For this review, take the finished solid that the model builds, in its own axes (mm). Face numbers are marked on the shaded views. A direction names the side the tool comes from. Give positions to 0.01 mm unless a question says otherwise; leave off trailing zeros. Order: outer loops, then holes, each group sorted by start corner. A loop starts at its lowest first (then second) coordinate and runs counter-clockwise, first axis right, second up. Notation, with made-up numbers: (-27, 65) - (9, 65) arc R15 ccw to (9, 85) - close; hole circle Ø5 at (43.5, 7.25). An arc over 180 degrees is marked (long way). Answer as a JSON object with one key per item and string values. Group by question number.
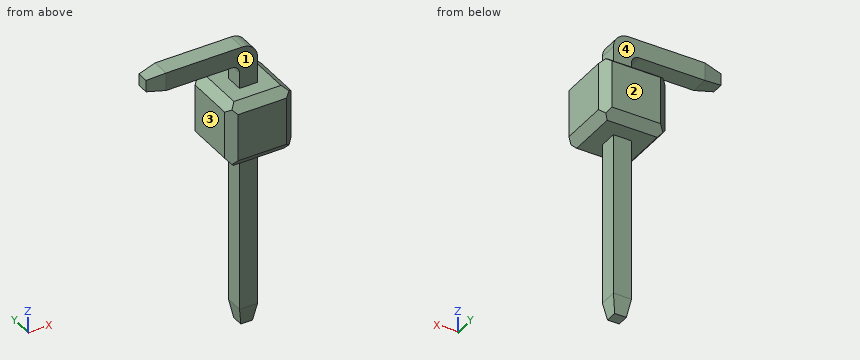
from build123d import *
from OCP.BRepFilletAPI import BRepFilletAPI_MakeChamfer

# Parameters (mm, degrees)
EXTRUDE_1_DEPTH = 0.7
CHAMFER_1_SIZE  = 0.7
CHAMFER_1_SIZE2 = 0.123428886
CHAMFER_2_SIZE  = 0.7
CHAMFER_2_SIZE2 = 0.123428886
SKETCH_2_W      = 2.54
SKETCH_2_H      = 2.54
EXTRUDE_2_DEPTH = 2.5
CHAMFER_3_SIZE  = 0.3
CHAMFER_3_SIZE2 = 0.357526078
CHAMFER_4_SIZE  = 0.3
CHAMFER_4_SIZE2 = 0.357526078
CHAMFER_5_SIZE  = 0.3
CHAMFER_5_SIZE2 = 0.357526078


with BuildPart() as part:
    # Эскиз1 → Бобышка-Вытянуть1 (new body)
    with BuildSketch(Plane(origin=(0, 0, 0), x_dir=(1, 0, 0), z_dir=(0, 1, 0))):
        with BuildLine():
            Line((0.35, 0), (0.35, -10.55))
            ThreePointArc((0.35, -10.55), (0.174264069, -10.974264069), (-0.25, -11.15))
            Line((-0.25, -11.15), (-3.9, -11.15))
            Line((-3.9, -11.15), (-3.9, -10.45))
            Line((-3.9, -10.45), (-0.65, -10.45))
            ThreePointArc((-0.65, -10.45), (-0.437867966, -10.362132034), (-0.35, -10.15))
            Line((-0.35, -10.15), (-0.35, 0))
            Line((-0.35, 0), (0.35, 0))
        make_face()
    extrude(amount=EXTRUDE_1_DEPTH)

    # Фаска1: one chamfer whose edges measure the first distance from different faces: ONE call of the kernel's chamfer builder (chamfer() names one face for all edges)
    chamfer_1_edges_1 = [part.edges().sort_by_distance(p)[0] for p in [
        (0, 0, 0),
    ]]
    chamfer_1_side_1 = [part.faces().sort_by_distance(p)[0] for p in [
        (-0.230674814, 0, 5.075),
    ]]
    chamfer_1_edges_2 = [part.edges().sort_by_distance(p)[0] for p in [
        (0.35, 0.35, 0),
    ]]
    chamfer_1_side_2 = [part.faces().sort_by_distance(p)[0] for p in [
        (0.35, 0.35, 5.275),
    ]]
    chamfer_1_edges_3 = [part.edges().sort_by_distance(p)[0] for p in [
        (-0.35, 0.35, 0),
    ]]
    chamfer_1_side_3 = [part.faces().sort_by_distance(p)[0] for p in [
        (-0.35, 0.35, 5.075),
    ]]
    chamfer_1_edges_4 = [part.edges().sort_by_distance(p)[0] for p in [
        (0, 0.7, 0),
    ]]
    chamfer_1_side_4 = [part.faces().sort_by_distance(p)[0] for p in [
        (-0.230674814, 0.7, 5.075),
    ]]
    chamfer_1 = BRepFilletAPI_MakeChamfer(part.part.solid().wrapped)
    for e in chamfer_1_edges_1:
        chamfer_1.Add(CHAMFER_1_SIZE, CHAMFER_1_SIZE2, e.wrapped, chamfer_1_side_1[0].wrapped)  # the first distance lies on this face
    for e in chamfer_1_edges_2:
        chamfer_1.Add(CHAMFER_1_SIZE, CHAMFER_1_SIZE2, e.wrapped, chamfer_1_side_2[0].wrapped)  # the first distance lies on this face
    for e in chamfer_1_edges_3:
        chamfer_1.Add(CHAMFER_1_SIZE, CHAMFER_1_SIZE2, e.wrapped, chamfer_1_side_3[0].wrapped)  # the first distance lies on this face
    for e in chamfer_1_edges_4:
        chamfer_1.Add(CHAMFER_1_SIZE, CHAMFER_1_SIZE2, e.wrapped, chamfer_1_side_4[0].wrapped)  # the first distance lies on this face
    add(Compound.cast(chamfer_1.Shape()), mode=Mode.REPLACE)

    # Фаска2: one chamfer whose edges measure the first distance from different faces: ONE call of the kernel's chamfer builder (chamfer() names one face for all edges)
    chamfer_2_edges_1 = [part.edges().sort_by_distance(p)[0] for p in [
        (-3.9, 0.35, 11.15),
    ]]
    chamfer_2_side_1 = [part.faces().sort_by_distance(p)[0] for p in [
        (-2.075, 0.35, 11.15),
    ]]
    chamfer_2_edges_2 = [part.edges().sort_by_distance(p)[0] for p in [
        (-3.9, 0.35, 10.45),
    ]]
    chamfer_2_side_2 = [part.faces().sort_by_distance(p)[0] for p in [
        (-2.275, 0.35, 10.45),
    ]]
    chamfer_2_edges_3 = [part.edges().sort_by_distance(p)[0] for p in [
        (-3.9, 0.7, 10.8),
    ]]
    chamfer_2_side_3 = [part.faces().sort_by_distance(p)[0] for p in [
        (-0.23718821, 0.7, 5.425),
    ]]
    chamfer_2_edges_4 = [part.edges().sort_by_distance(p)[0] for p in [
        (-3.9, 0, 10.8),
    ]]
    chamfer_2_side_4 = [part.faces().sort_by_distance(p)[0] for p in [
        (-0.23718821, 0, 5.425),
    ]]
    chamfer_2 = BRepFilletAPI_MakeChamfer(part.part.solid().wrapped)
    for e in chamfer_2_edges_1:
        chamfer_2.Add(CHAMFER_2_SIZE, CHAMFER_2_SIZE2, e.wrapped, chamfer_2_side_1[0].wrapped)  # the first distance lies on this face
    for e in chamfer_2_edges_2:
        chamfer_2.Add(CHAMFER_2_SIZE, CHAMFER_2_SIZE2, e.wrapped, chamfer_2_side_2[0].wrapped)  # the first distance lies on this face
    for e in chamfer_2_edges_3:
        chamfer_2.Add(CHAMFER_2_SIZE, CHAMFER_2_SIZE2, e.wrapped, chamfer_2_side_3[0].wrapped)  # the first distance lies on this face
    for e in chamfer_2_edges_4:
        chamfer_2.Add(CHAMFER_2_SIZE, CHAMFER_2_SIZE2, e.wrapped, chamfer_2_side_4[0].wrapped)  # the first distance lies on this face
    add(Compound.cast(chamfer_2.Shape()), mode=Mode.REPLACE)

    # Эскиз2 → Бобышка-Вытянуть2 (add)
    with BuildSketch(Plane.XY.offset(9.53)):
        with Locations((0, 0.35)):
            Rectangle(SKETCH_2_W, SKETCH_2_H)
    extrude(amount=-EXTRUDE_2_DEPTH)

    # Фаска3
    chamfer_3_edges = [part.edges().sort_by_distance(p)[0] for p in [
        (-1.27, 0.35, 7.03),
        (0, 1.62, 7.03),
        (1.27, 0.35, 7.03),
        (0, -0.92, 7.03),
    ]]
    chamfer_3_side = [part.faces().sort_by_distance(p)[0] for p in [
        (0, -0.884078976, 7.03),
    ]]
    chamfer(chamfer_3_edges, length=CHAMFER_3_SIZE, length2=CHAMFER_3_SIZE2, reference=chamfer_3_side[0])

    # Фаска4: one chamfer whose edges measure the first distance from different faces: ONE call of the kernel's chamfer builder (chamfer() names one face for all edges)
    chamfer_4_edges_1 = [part.edges().sort_by_distance(p)[0] for p in [
        (-1.27, 0.35, 9.53),
    ]]
    chamfer_4_side_1 = [part.faces().sort_by_distance(p)[0] for p in [
        (-1.27, 0.35, 8.458763039),
    ]]
    chamfer_4_edges_2 = [part.edges().sort_by_distance(p)[0] for p in [
        (0, -0.92, 9.53),
    ]]
    chamfer_4_side_2 = [part.faces().sort_by_distance(p)[0] for p in [
        (0, -0.92, 8.458763039),
    ]]
    chamfer_4_edges_3 = [part.edges().sort_by_distance(p)[0] for p in [
        (1.27, 0.35, 9.53),
    ]]
    chamfer_4_side_3 = [part.faces().sort_by_distance(p)[0] for p in [
        (1.27, 0.35, 8.458763039),
    ]]
    chamfer_4_edges_4 = [part.edges().sort_by_distance(p)[0] for p in [
        (0, 1.62, 9.53),
    ]]
    chamfer_4_side_4 = [part.faces().sort_by_distance(p)[0] for p in [
        (0, 1.62, 8.458763039),
    ]]
    chamfer_4 = BRepFilletAPI_MakeChamfer(part.part.solid().wrapped)
    for e in chamfer_4_edges_1:
        chamfer_4.Add(CHAMFER_4_SIZE, CHAMFER_4_SIZE2, e.wrapped, chamfer_4_side_1[0].wrapped)  # the first distance lies on this face
    for e in chamfer_4_edges_2:
        chamfer_4.Add(CHAMFER_4_SIZE, CHAMFER_4_SIZE2, e.wrapped, chamfer_4_side_2[0].wrapped)  # the first distance lies on this face
    for e in chamfer_4_edges_3:
        chamfer_4.Add(CHAMFER_4_SIZE, CHAMFER_4_SIZE2, e.wrapped, chamfer_4_side_3[0].wrapped)  # the first distance lies on this face
    for e in chamfer_4_edges_4:
        chamfer_4.Add(CHAMFER_4_SIZE, CHAMFER_4_SIZE2, e.wrapped, chamfer_4_side_4[0].wrapped)  # the first distance lies on this face
    add(Compound.cast(chamfer_4.Shape()), mode=Mode.REPLACE)

    # Фаска5: one chamfer whose edges measure the first distance from different faces: ONE call of the kernel's chamfer builder (chamfer() names one face for all edges)
    chamfer_5_edges_1 = [part.edges().sort_by_distance(p)[0] for p in [
        (-1.27, -0.92, 8.308763039),
    ]]
    chamfer_5_side_1 = [part.faces().sort_by_distance(p)[0] for p in [
        (0, -0.92, 8.308763039),
    ]]
    chamfer_5_edges_2 = [part.edges().sort_by_distance(p)[0] for p in [
        (1.27, -0.92, 8.308763039),
    ]]
    chamfer_5_side_2 = [part.faces().sort_by_distance(p)[0] for p in [
        (1.27, 0.35, 8.308763039),
    ]]
    chamfer_5_edges_3 = [part.edges().sort_by_distance(p)[0] for p in [
        (-1.27, 1.62, 8.308763039),
    ]]
    chamfer_5_side_3 = [part.faces().sort_by_distance(p)[0] for p in [
        (-1.27, 0.35, 8.308763039),
    ]]
    chamfer_5_edges_4 = [part.edges().sort_by_distance(p)[0] for p in [
        (1.27, 1.62, 8.308763039),
    ]]
    chamfer_5_side_4 = [part.faces().sort_by_distance(p)[0] for p in [
        (0, 1.62, 8.308763039),
    ]]
    chamfer_5 = BRepFilletAPI_MakeChamfer(part.part.solid().wrapped)
    for e in chamfer_5_edges_1:
        chamfer_5.Add(CHAMFER_5_SIZE, CHAMFER_5_SIZE2, e.wrapped, chamfer_5_side_1[0].wrapped)  # the first distance lies on this face
    for e in chamfer_5_edges_2:
        chamfer_5.Add(CHAMFER_5_SIZE, CHAMFER_5_SIZE2, e.wrapped, chamfer_5_side_2[0].wrapped)  # the first distance lies on this face
    for e in chamfer_5_edges_3:
        chamfer_5.Add(CHAMFER_5_SIZE, CHAMFER_5_SIZE2, e.wrapped, chamfer_5_side_3[0].wrapped)  # the first distance lies on this face
    for e in chamfer_5_edges_4:
        chamfer_5.Add(CHAMFER_5_SIZE, CHAMFER_5_SIZE2, e.wrapped, chamfer_5_side_4[0].wrapped)  # the first distance lies on this face
    add(Compound.cast(chamfer_5.Shape()), mode=Mode.REPLACE)


solid = part.part
1) Consider section B-B (x = -2.2). Give the boundary of the cut face in (y, z).
2) For line 1 (X direction, y = -0.3, z = 8.25); line 2 (Y direction, x = 0.3, z = 4.75); line 3 (Z direction, x = 0.25, y = -0.55), list the stretches that pass through material, from the lowest coordinate up.
3) For the marked faces 1, 2, 3 and 4, list the 3-axis set-ups (+Z, -Z, +X, -X, +Y, -Y) from which the entire face can be reached by the end or side of a thin tool; tool diameter is ignored.
4) For pin 1 (0.8 mm diameter, centred on y = 0.5, z = 2.5, fed in from -X); pin 2 (0.8 mm diameter, centred on x = 0, z = 5.5, fed in from -Y); pin 3 (0.8 mm diameter, centred on y = 0.5, z = 10, fed in from +X), all flat-tipped, find the tip position at first contact; note any pin that passes through.
5) Consider section C-C (z = 6.75). Give the boundary of the cut face in (x, y).
6) Consider section A-A (y = 0.3). Give the boundary of the cut face in (x, z).
Result set:
{
 "1": {"outline": "(0, 10.45) - (0.7, 10.45) - (0.7, 11.15) - (0, 11.15) - close"},
 "2": {"line 1": "x = -1.27 to 1.27", "line 2": "y = 0 to 0.7", "line 3": "z = 7.03 to 9.53"},
 "3": {"face 1": "+Z, +X, -X, -Y", "face 2": "+Z, -Z, +X, -X, +Y", "face 3": "-Z, -X, +Y, -Y", "face 4": "+Z, +X, -X, +Y"},
 "4": {"pin 1": "stops at x = -0.35", "pin 2": "stops at y = 0", "pin 3": "stops at x = 0.35"},
 "5": {"outline": "(-0.35, 0) - (0.35, 0) - (0.35, 0.7) - (-0.35, 0.7) - close"},
 "6": {"outline": "(-3.9, 10.57) - (-3.2, 10.45) - (-0.65, 10.45) arc R0.3 cw to (-0.35, 10.15) - (-0.35, 9.53) - (-0.91, 9.53) - (-1.27, 9.23) - (-1.27, 7.39) - (-0.97, 7.03) - (-0.35, 7.03) - (-0.35, 0.7) - (-0.23, 0) - (0.23, 0) - (0.35, 0.7) - (0.35, 7.03) - (0.97, 7.03) - (1.27, 7.39) - (1.27, 9.23) - (0.91, 9.53) - (0.35, 9.53) - (0.35, 10.55) arc R0.6 ccw to (-0.25, 11.15) - (-3.2, 11.15) - (-3.9, 11.03) - close"}
}
